from build123d import *

# Parameters (mm, degrees)
SKETCH1_R           = 1.8
BOSS_EXTRUDE1_DEPTH = 3
FILLET2_R           = 5
FILLET3_R           = 3


with BuildPart() as part:
    # Sketch1 → Boss-Extrude1 (new body)
    with BuildSketch(Plane.XY):
        with BuildLine():
            Line((4.330127019, 2.5), (9.814954576, -7))
            Line((9.814954576, -7), (23.5, -7))
            Line((23.5, -7), (23.5, 5))
            ThreePointArc((23.5, 5), (28.5, 10), (33.5, 5))
            Line((33.5, 5), (33.5, -17))
            Line((33.5, -17), (4.041451884, -17))
            Line((4.041451884, -17), (-4.330127019, -2.5))
            ThreePointArc((-4.330127019, -2.5), (-2.5, 4.330127019), (4.330127019, 2.5))
        make_face()
        Circle(SKETCH1_R, mode=Mode.SUBTRACT)
    extrude(amount=BOSS_EXTRUDE1_DEPTH)

    # Fillet2
    fillet2_edges = [part.edges().sort_by_distance(p)[0] for p in [
        (33.5, -17, 1.5),
        (4.041451884, -17, 1.5),
    ]]
    fillet(fillet2_edges, radius=FILLET2_R)

    # Fillet3
    fillet3_edges = [part.edges().sort_by_distance(p)[0] for p in [
        (9.814954576, -7, 1.5),
        (23.5, -7, 1.5),
    ]]
    fillet(fillet3_edges, radius=FILLET3_R)


solid = part.part
Geometry: final body of the model. Coordinates: model frame, mm. A direction names the side the tool comes from. Round coordinates to 2 decimals unless told otherwise and drop trailing zeros. Order: outer loops, then holes, each group sorted by start corner. A loop starts at its lowest first (then second) coordinate and runs counter-clockwise, first axis right, second up. Notation, with made-up numbers: (-39, 86.5) -> (-30, 86.5) arc R21 cw to (-30, 91.5) -> close; hole circle Ø4 at (36.25, 37). An arc over 180 degrees is marked (long way). Put each result on its own line as item: value. Start each with the question number.
Q1. Section C-C on y = 0. Return the cut outline in (x, z).
Q2. Reachability of faces 5 (the flat face through (23.5, 0, 1)), 6 (the flat face through (19, -9, 3)) from +Z, -Z, +X, -X, +Y, -Y: full face, straight path, thin tool, end or side. Return the list, or none.
Q3. Section A-A on x = 0. Return the cut outline in (y, z), and give its area (3 significant figures).
Q4. First-contact query: pin 1 (1.5 mm diameter, centred on x = 17.5, z = 1.5, fed in from +Y); pin 2 (3 mm diameter, centred on x = 0, y = 0, fed in from -Z). Flat tips, straight axial feed; report the tip coordinate or a pass-through.
Q5. Pull-direction query (X, two-part tool) for faces 1 (the cylindrical face through (32, -15.57, 1.52)), 2 (the cylindrical face through (4.397, -16.312, 1.521)), 3 (the cylindrical face through (28.4, 10, 1.5)), 4 (the cylindrical face through (22.6, -6.14, 1.52)); classes: +X half, -X half, draft (parallel to the pull), parting line (faces both ways), or undercut.
Q6. Section D-D on y = -5. Return the cut outline in (x, z), and give its area (3 significant figures).
Q7. Line query: probe 1 along Y at (x, z) = (19, 1.9); probe 2 along Y at (x, z) = (-0.5, 1.05); probe 3 along X at (y, z) = (3.5, 0.2). Output: solid intervals per line, ascending.
Q8. Section B-B on z = 1.05. Return the cut outline in (x, y).
Ans:
1. outline: (-5, 0) -> (-1.8, 0) -> (-1.8, 3) -> (-5, 3) -> close; (1.8, 0) -> (5.77, 0) -> (5.77, 3) -> (1.8, 3) -> close; (23.5, 0) -> (33.5, 0) -> (33.5, 3) -> (23.5, 3) -> close
2. face 5: +Z, -Z, +Y
2. face 6: +Z, +X, -X, +Y, -Y
3. outline: (-10, 0) -> (-1.8, 0) -> (-1.8, 3) -> (-10, 3) -> close; (1.8, 0) -> (5, 0) -> (5, 3) -> (1.8, 3) -> close
3. area: 34.2 mm2
4. pin 1: stops at y = -7
4. pin 2: passes through
5. face 1: +X half
5. face 2: -X half
5. face 3: parting line
5. face 4: undercut
6. outline: (-2.89, 0) -> (8.66, 0) -> (8.66, 3) -> (-2.89, 3) -> close; (23.33, 0) -> (33.5, 0) -> (33.5, 3) -> (23.33, 3) -> close
6. area: 65.2 mm2
7. probe 1: y = -17 to -7
7. probe 2: y = -9.13 to -1.73, 1.73 to 4.97
7. probe 3: x = -3.57 to 3.57, 23.5 to 33.5
8. outline: (-4.33, -2.5) -> (2.6, -14.5) arc R5 ccw to (6.93, -17) -> (28.5, -17) arc R5 ccw to (33.5, -12) -> (33.5, 5) arc R5 ccw to (23.5, 5) -> (23.5, -4) arc R3 cw to (20.5, -7) -> (11.55, -7) arc R3 cw to (8.95, -5.5) -> (4.33, 2.5) arc R5 ccw to start; hole circle Ø3.6 at (0, 0)
